Verification items for the finished model (mm, model axes). Round coordinates to 2 decimals unless told otherwise and drop trailing zeros. Write each loop counter-clockwise with the first axis right and the second up, starting at its lowest first coordinate (ties: lowest second). Pieces come first, ordered by that corner, then holes.
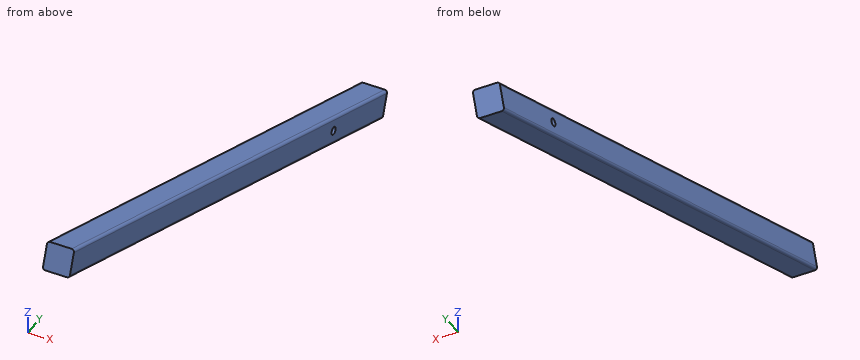
from build123d import *

# Parameters (mm, degrees)
SKETCH1_W                  = 30
SKETCH1_H                  = 700
BOSS_EXTRUDE1_DEPTH        = 30
F_8_5_8_5_DIAMETER_HOLE1_D = 8.5
FILLET1_R                  = 3


with BuildPart() as part:
    # Sketch1 → Boss-Extrude1 (new body)
    with BuildSketch(Plane(origin=(0, 581.941084715, 1587.910176451), x_dir=(-1, 0, 0), z_dir=(0, 0.3441021099188428, 0.9389322328844616))):
        with Locations((13.69090897, 276.656236502)):
            Rectangle(SKETCH1_W, SKETCH1_H)
    extrude(amount=-BOSS_EXTRUDE1_DEPTH)

    # Ø8.5 (8.5) Diameter Hole1 (through all)
    with Locations(Plane(origin=(1.30909103, 0, 0), x_dir=(0, 0, -1), z_dir=(1, 0, 0))):
        with Locations((-1588.160191829, 537.667169913)):
            Hole(F_8_5_8_5_DIAMETER_HOLE1_D / 2)

    # Fillet1
    fillet1_edges = [part.edges().sort_by_distance(p)[0] for p in [
        (1.30909103, 311.856563537, 1654.940204167),
        (-28.69090897, 311.856563537, 1654.940204167),
        (1.30909103, 322.179626834, 1683.108171153),
        (-28.69090897, 322.179626834, 1683.108171153),
    ]]
    fillet(fillet1_edges, radius=FILLET1_R)


solid = part.part
Q1. Depth check by flat-ended pin: P1, Ø2, axis at x = -9.5, z = 1562, coming from the +Y side; P2, Ø3, axis at x = -22, y = 192.5, coming from the -Z side; P3, Ø8, axis at x = -20, y = 362, coming from the -Z side. Enter the tip coordinate at first touch or a pass-through.
Recorded:
P1: stops at y = 650.81
P2: stops at z = 1698.13
P3: stops at z = 1635.1
Q2. Sectioned sample at A-A (x = -14). Enter the section's corners in (y, z).
Recorded:
outline: (-16.77, 1775.38) - (640.48, 1534.5) - (650.81, 1562.67) - (-6.45, 1803.54) - close; hole circle Ø8.5 at (537.67, 1588.16)
Q3. Material ranges on line 1 along Z through (x, y) = (-2, 107.5); line 2 along Z through (x, y) = (-5.5, 143), recorded low to high.
Recorded:
line 1: z = 1729.83 to 1761.78
line 2: z = 1716.82 to 1748.77
